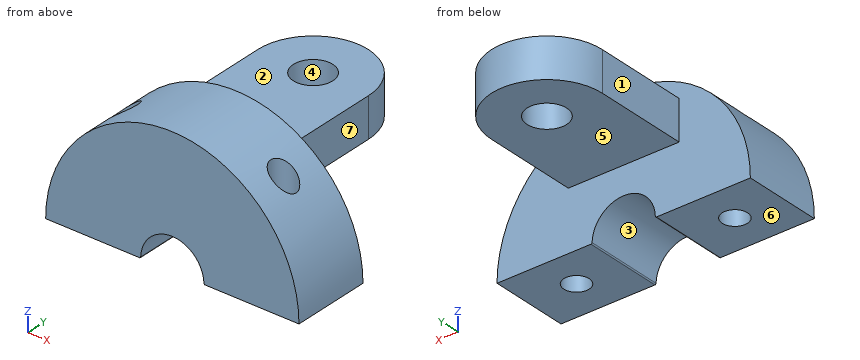
```python
from build123d import *

# Parameters (mm, degrees)
BOSS_EXTRUDE1_DEPTH   = 2.5
SKETCH2_W             = 7
SKETCH2_H             = 2.5
BOSS_EXTRUDE2_DEPTH   = 9.5
CUT_EXTRUDE1_DEPTH    = 9.5
SKETCH4_R             = 1.25
CUT_EXTRUDE2_DEPTH    = 9.5
M2X0_4_TAPPED_HOLE1_D = 1.6
FILLET1_R             = 0.07


with BuildPart() as part:
    # Sketch1 → Boss-Extrude1 (new body, symmetric)
    with BuildSketch(Plane(origin=(0, 0, 0), x_dir=(1, 0, 0), z_dir=(0, 1, 0))):
        with BuildLine():
            Line((2, 0), (8, 0))
            ThreePointArc((8, 0), (0, -8), (-8, 0))
            Line((-8, 0), (-2, 0))
            ThreePointArc((-2, 0), (0, -2), (2, 0))
        make_face()
    extrude(amount=BOSS_EXTRUDE1_DEPTH, both=True)

    # Sketch2 → Boss-Extrude2 (add)
    with BuildSketch(Plane(origin=(0, 2.5, 0), x_dir=(1, 0, 0), z_dir=(0, 1, 0))):
        with Locations((0, -5)):
            Rectangle(SKETCH2_W, SKETCH2_H)
    extrude(amount=BOSS_EXTRUDE2_DEPTH)

    # Sketch3 → Cut-Extrude1 (cut)
    with BuildSketch(Plane(origin=(0, 0, 3.75), x_dir=(-1, 0, 0), z_dir=(0, 0, -1))):
        with BuildLine():
            Line((-3.5, 8.5), (-3.5, 14.886359519))
            Line((-3.5, 14.886359519), (0, 16.809201746))
            Line((0, 16.809201746), (3.5, 14.5))
            Line((3.5, 14.5), (3.5, 8.5))
            ThreePointArc((3.5, 8.5), (0, 12), (-3.5, 8.5))
        make_face()
    extrude(amount=-CUT_EXTRUDE1_DEPTH, mode=Mode.SUBTRACT)

    # Sketch4 → Cut-Extrude2 (cut)
    with BuildSketch(Plane(origin=(0, 0, 3.75), x_dir=(-1, 0, 0), z_dir=(0, 0, -1))):
        with Locations((0, 8.5)):
            Circle(SKETCH4_R)
    extrude(amount=-CUT_EXTRUDE2_DEPTH, mode=Mode.SUBTRACT)

    # M2x0.4 Tapped Hole1 (through all)
    with Locations(Plane(origin=(0, 0, 0), x_dir=(-1, 0, 0), z_dir=(0, 0, -1))):
        with Locations((-5, 0), (5, 0)):
            Hole(M2X0_4_TAPPED_HOLE1_D / 2)

    # Fillet1
    fillet1_edges = [part.edges().sort_by_distance(p)[0] for p in [
        (2, 0, 0),
        (-2, 0, 0),
    ]]
    fillet(fillet1_edges, radius=FILLET1_R)


solid = part.part
```
Source: CAD feature listing. Evaluate the final solid. Frame: model axes, mm. Face numbers are marked on the shaded views. A direction names the side the tool comes from. Coordinates: 2 decimals unless noted, no trailing zeros. Write each loop counter-clockwise with the first axis right and the second up, starting at its lowest first coordinate (ties: lowest second). Pieces come first, ordered by that corner, then holes. Notation, with made-up numbers: M -34,49.25 L -4,49.25 A28 ccw -4,87.25 Z; hole C 68.5,-26.75 d3. An arc over 180 degrees is marked long. Answer as a JSON object with one key per item and string values.
1. Cut plane A-A on x = 0. Output: boundary loops of the cut face in (y, z).
Evaluation:
{"outline": "M -2.5,2 L 2.5,2 L 2.5,3.75 L 7.25,3.75 L 7.25,6.25 L 2.5,6.25 L 2.5,8 L -2.5,8 Z; M 9.75,3.75 L 12,3.75 L 12,6.25 L 9.75,6.25 Z"}
2. Access query for the marked faces 5, 6 and 7. Directions: +Z, -Z, +X, -X, +Y, -Y. A direction counts if a zero-diameter tool reaches every point of the face in a straight line with its end or side. Return the directions, or none.
Evaluation:
{"face 5": "-Z, +X, -X, +Y", "face 6": "-Z, +X, -X, +Y, -Y", "face 7": "+Z, -Z, +X, +Y"}
3. Cut plane D-D on x = 5. Output: boundary loops of the cut face in (y, z) (3 decimals).
Evaluation:
{"outline": "M -2.5,0 L -0.8,0 L -0.8,6.245 L -2.5,6.245 Z; M 0.8,0 L 2.5,0 L 2.5,6.245 L 0.8,6.245 Z"}
4. Cut plane C-C on z = 2.5. Output: boundary loops of the cut face in (x, y).
Evaluation:
{"outline": "M -7.6,-2.5 L 7.6,-2.5 L 7.6,2.5 L -7.6,2.5 Z; hole C -5,0 d1.6; hole C 5,0 d1.6"}
5. Cut plane B-B on z = 4.75. Output: boundary loops of the cut face in (x, y).
Evaluation:
{"outline": "M -6.44,-2.5 L 6.44,-2.5 L 6.44,2.5 L 3.5,2.5 L 3.5,8.5 A3.5 ccw -3.5,8.5 L -3.5,2.5 L -6.44,2.5 Z; hole C -5,0 d1.6; hole C 0,8.5 d2.5; hole C 5,0 d1.6"}
6. Contact query for flat-ended pins moving along their axis: P1, Ø7.5, axis at x = 0.5, y = 7, coming from the +Z side; P2, Ø1, axis at y = 4, z = 5.5, coming from the +X side; P3, Ø5.5, axis at x = -1, y = 7.5, coming from the -Z side. Output: stop coordinate, or through.
Evaluation:
{"P1": "z = 6.25", "P2": "x = 3.5", "P3": "z = 3.75"}
7. Ray query, L1, parallel to Y at x = -5, z = 2; L2, parallel to X at y = 0.5, z = 3.25; L3, parallel to Z at x = 1, y = 11.25. Return the intervals inside material, ascending.
Evaluation:
{"L1": "-2.5 to -0.8, 0.8 to 2.5", "L2": "-7.31 to -5.62, -4.38 to 4.38, 5.62 to 7.31", "L3": "3.75 to 6.25"}
8. Draft query along X for the marked faces 1, 2, 3 and 4. Return one class per face: released by +X, released by -X, zero draft, split by the parting line, or undercut.
Evaluation:
{"face 1": "released by -X", "face 2": "zero draft", "face 3": "undercut", "face 4": "undercut"}
